from build123d import *

# Parameters (mm, degrees)
EXTRUDE_1_DEPTH     = 10
SKETCH_3_W          = 5
SKETCH_3_H          = 16.2
CUT_EXTRUDE_1_DEPTH = 8.5


with BuildPart() as part:
    # Эскиз2 → Бобышка-Вытянуть1 (new body)
    with BuildSketch(Plane.XY):
        with BuildLine():
            Line((-2.5, 8.1), (-11, 8.1))
            ThreePointArc((-11, 8.1), (0, 13.660527076), (11, 8.1))
            Line((11, 8.1), (2.5, 8.1))
            Line((2.5, 8.1), (2.5, -8.1))
            Line((2.5, -8.1), (11, -8.1))
            ThreePointArc((11, -8.1), (0, -13.660527076), (-11, -8.1))
            Line((-11, -8.1), (-2.5, -8.1))
            Line((-2.5, -8.1), (-2.5, 8.1))
        make_face()
    extrude(amount=EXTRUDE_1_DEPTH)

    # Эскиз3 → Вырез-Вытянуть1 (cut)
    with BuildSketch(Plane.XY.offset(10)):
        Rectangle(SKETCH_3_W, SKETCH_3_H)
    extrude(amount=-CUT_EXTRUDE_1_DEPTH, mode=Mode.SUBTRACT)


solid = part.part
Source: CAD feature listing. Evaluate the final solid. Frame: model axes, mm. A direction names the side the tool comes from. Give positions to 0.01 mm unless a question says otherwise; leave off trailing zeros. Write each loop counter-clockwise with the first axis right and the second up, starting at its lowest first coordinate (ties: lowest second). Pieces come first, ordered by that corner, then holes. Notation, with made-up numbers: (-34.75, 38) - (-16.75, 38) arc R16 cw to (-16.75, 59) - close; hole circle Ø9 at (21, 28.25). An arc over 180 degrees is marked (long way). Write item = value, one per line. Start each with the question number.
Q1. Cut plane B-B, the plane z = 8.75. Return loops of the section in (x, y).
Q2. Cut plane C-C, the plane z = 1. Return loops of the section in (x, y), then the cut area to 3 significant figures.
Q3. Material intervals for probe 1 along Y at (x, z) = (0, 8.5); probe 2 along Y at (x, z) = (2.5, 8); probe 3 along Z at (x, y) = (0.5, -4.75), sorted ascending.
Q4. Cut plane A-A, the plane x = 4.75. Return loops of the section in (y, z), then the cut area to 3 significant figures.
Q5. Pin query (flat end, axial travel): pin 1 Ø0.8 at (y, z) = (-1, 1) entering from -X; pin 2 Ø2 at (x, z) = (7, 6) entering from +Y; pin 3 Ø3 at (x, z) = (7.5, 8.5) entering from -Y. Return the tip coordinate at first contact, or that it passes through.
Q6. Cut plane D-D, the plane y = 11. Return loops of the section in (x, z).
Q7. Reachability of faces 1 (the flat face through (0, 0, 1.5)), 2 (the flat face through (2.5, 0, 1)), 3 (the flat face through (-2.5, 0, 1)) from +Z, -Z, +X, -X, +Y, -Y: full face, straight path, thin tool, end or side. Return the list, or none.
Q8. Draft query along Y for faces 4 (the flat face through (0, -8.1, 5)), 5 (the flat face through (0, 10, 10)), 6 (the cylindrical face through (-0.18, 13.66, 4.93)). Return one class per face: +Y half, -Y half, draft (parallel to the pull), parting line (faces both ways), or undercut.
Computed values:
q1.outline = (-11, -8.1) arc R13.66 ccw to (11, -8.1) - close; (-11, 8.1) - (11, 8.1) arc R13.66 ccw to start
q2.outline = (-11, -8.1) arc R13.66 ccw to (11, -8.1) - (2.5, -8.1) - (2.5, 8.1) - (11, 8.1) arc R13.66 ccw to (-11, 8.1) - (-2.5, 8.1) - (-2.5, -8.1) - close
q2.area = 252 mm²
q3.probe_1 = -13.66 to -8.1, 8.1 to 13.66
q3.probe_2 = -13.43 to -8.1, 8.1 to 13.43
q3.probe_3 = 0 to 1.5
q4.outline = (-12.81, 0) - (-8.1, 0) - (-8.1, 10) - (-12.81, 10) - close; (8.1, 0) - (12.81, 0) - (12.81, 10) - (8.1, 10) - close
q4.area = 94.2 mm²
q5.pin_1 = -2.5
q5.pin_2 = 12.27
q5.pin_3 = -12.27
q6.outline = (-8.1, 0) - (8.1, 0) - (8.1, 10) - (-8.1, 10) - close
q7.face_1 = +Z, +X, -X
q7.face_2 = +Z, -Z, +X
q7.face_3 = +Z, -Z, -X
q8.face_4 = undercut
q8.face_5 = draft
q8.face_6 = +Y half
